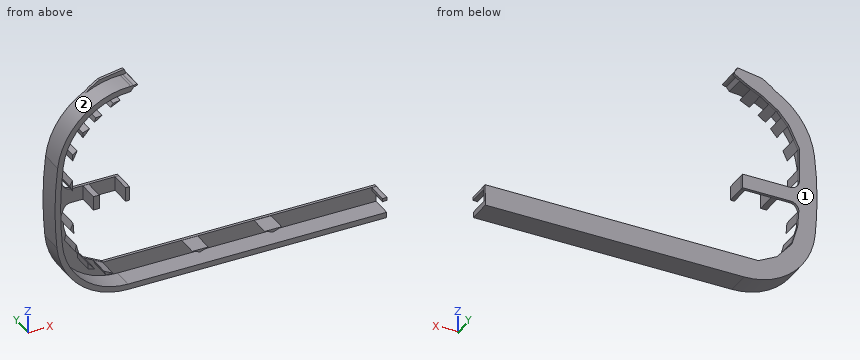
```python
from build123d import *

# Parameters (mm, degrees)
PAD356_DEPTH  = 12.5
PAD357_DEPTH  = 1.5
SKETCH835_W   = 2.131072
SKETCH835_H   = 7.619457
SKETCH835_W_2 = 3.147286
SKETCH835_H_2 = 7.516819
PAD359_DEPTH  = 11


with BuildPart() as part:
    # Sketch830 → Pad356 (new body)
    with BuildSketch(Plane.XZ):
        with BuildLine():
            Line((-1.478534, -110.025169), (137.370667, -110.025169))
            Line((137.370667, -107.025169), (137.370667, -110.025169))
            Line((-1.431571, -107.025169), (137.370667, -107.025169))
            ThreePointArc((-36.592097, -75.335952), (-25.110465, -97.94725), (-1.431571, -107.025169))
            ThreePointArc((-36.186878, -30.666211), (-37.587109, -52.990217), (-36.592097, -75.335952))
            ThreePointArc((0, 1.374966), (-24.161208, -7.792765), (-36.186878, -30.666211))
            Line((1.544739, 3.529825), (0, 1.374966))
            ThreePointArc((1.544739, 3.529825), (2.72516, 3.732882), (3.781105, 4.298219))
            Line((3.239563, 4.948117), (3.781105, 4.298219))
            ThreePointArc((1.508208, 4.37461), (2.420143, 4.521718), (3.239563, 4.948117))
            Line((0.022068, 4.37461), (1.508208, 4.37461))
            ThreePointArc((0.022068, 4.37461), (-26.243945, -5.630658), (-39.196845, -30.575221))
            ThreePointArc((-39.196845, -30.575221), (-40.587676, -52.998313), (-39.596378, -75.442618))
            ThreePointArc((-39.596378, -75.442618), (-27.212376, -100.091175), (-1.478534, -110.025169))
        make_face()
    extrude(amount=PAD356_DEPTH)

    # Sketch831 → Pad357 (join)
    with BuildSketch(Plane.XZ):
        with BuildLine():
            Line((-11.20697, 4.995917), (2.081055, 7.171183))
            Line((2.081055, 7.171183), (3.884949, 3.346928))
            Line((3.884949, 3.346928), (-3.071976, -0.758803))
            Line((-3.071976, -0.758803), (-10.956131, -4.609589))
            Line((-10.956131, -4.609589), (-19.896614, -10.750674))
            Line((-19.896614, -10.750674), (-25.51712, -17.174105))
            Line((-25.51712, -17.174105), (-31.174488, -28.94161))
            Line((-31.174488, -28.94161), (-31.174488, -40.845127))
            Line((-31.174488, -40.845127), (-31.174488, -47.004086))
            ThreePointArc((-31.174488, -47.004086), (-29.668559, -50.63972), (-26.032925, -52.145649))
            Line((-26.032925, -52.145649), (-0.596695, -52.145649))
            Line((-0.596695, -52.145649), (-0.596695, -59.85376))
            Line((-0.596695, -59.85376), (-26.454301, -59.85376))
            ThreePointArc((-26.454301, -59.85376), (-29.668775, -61.254046), (-30.832452, -64.561539))
            Line((-30.832452, -64.561539), (-30.207592, -73.162094))
            Line((-30.207592, -73.162094), (-27.154285, -83.944923))
            Line((-27.154285, -83.944923), (-18.964409, -93.499779))
            Line((-18.964409, -93.499779), (-9.168678, -98.558228))
            Line((-9.168678, -98.558228), (-2.331345, -98.558228))
            Line((-2.331345, -98.558228), (137.626465, -98.558228))
            Line((137.626465, -98.558228), (137.14772, -109.564461))
            Line((137.14772, -109.564461), (2.745987, -109.564461))
            Line((2.745987, -109.564461), (-3.35627, -109.564461))
            Line((-3.35627, -109.564461), (-8.527748, -108.903885))
            Line((-8.527748, -108.903885), (-14.660988, -106.811363))
            Line((-14.660988, -106.811363), (-18.737785, -105.296097))
            Line((-18.737785, -105.296097), (-23.031059, -102.842796))
            Line((-23.031059, -102.842796), (-25.966358, -100.308403))
            Line((-25.966358, -100.308403), (-29.71846, -96.772774))
            Line((-29.71846, -96.772774), (-33.867416, -91.108543))
            Line((-33.867416, -91.108543), (-35.409092, -87.704582))
            Line((-35.409092, -87.704582), (-37.577, -82.887016))
            Line((-37.577, -82.887016), (-39.02227, -76.142418))
            Line((-39.02227, -76.142418), (-39.504028, -68.916061))
            Line((-39.504028, -68.916061), (-39.795753, -62.945045))
            Line((-39.795753, -62.945045), (-39.795753, -54.118259))
            Line((-39.795753, -54.118259), (-39.795753, -44.679527))
            Line((-39.795753, -44.679527), (-38.558964, -32.354319))
            Line((-38.558964, -32.354319), (-38.395519, -29.4237))
            Line((-38.395519, -29.4237), (-36.619396, -22.319212))
            Line((-36.619396, -22.319212), (-33.174793, -14.730327))
            Line((-33.174793, -14.730327), (-28.806725, -8.890129))
            Line((-28.806725, -8.890129), (-22.724854, -3.669405))
            Line((-22.724854, -3.669405), (-15.835655, 1.92807))
            Line((-15.835655, 1.92807), (-11.20697, 4.995917))
        make_face()
    extrude(amount=PAD357_DEPTH)

    # Sketch835 → Pad359 (join)
    with BuildSketch(Plane.XZ.offset(1.5)):
        Polygon((-10.797218, -4.39096), (-5.61734, -1.866684), (-9.447662, -2.509944), align=None)
        Polygon((-19.402313, -10.356634), (-15.412445, -7.539076), (-18.804184, -8.036141), align=None)
        Polygon((-25.540901, -17.185297), (-22.080704, -13.161652), (-25.735592, -14.506651), align=None)
        Polygon((-28.749714, -23.759703), (-31.132679, -28.766081), (-31.176563, -25.309376), align=None)
        Polygon((-31.262688, -39.822292), (-31.262688, -45.629166), (-32.695404, -42.60001), align=None)
        with Locations((-1.667923, -55.987685)):
            Rectangle(SKETCH835_W, SKETCH835_H)
        with Locations((-18.408268, -55.977922)):
            Rectangle(SKETCH835_W_2, SKETCH835_H_2)
        Polygon((-30.88335, -63.977547), (-30.474003, -69.971565), (-32.403786, -67.427757), align=None)
        Polygon((-29.178089, -76.970978), (-27.78371, -82.030663), (-29.80479, -80.196259), align=None)
        Polygon((-23.049667, -88.872955), (-19.251656, -93.215378), (-22.826111, -92.215782), align=None)
        Polygon((-14.334663, -95.893806), (-9.420021, -98.582397), (-13.340538, -98.320648), align=None)
        Polygon((33.074181, -98.633934), (41.61673, -98.633934), (37.240623, -100.138222), align=None)
        Polygon((71.901031, -98.722458), (81.025146, -98.722458), (76.512283, -100.363495), align=None)
        Polygon((135.082978, -98.65696), (135.205872, -100.520859), (137.438461, -100.254593), (137.540878, -98.656967), align=None)
    extrude(amount=PAD359_DEPTH)


with BuildPart() as part_1:
    # Body024 placement: moved
    add(part.part.moved(Location((88, -111, 4))))


solid = part_1.part
```
Geometry check sheet. Reference: the model listing, model coordinates, mm. Face numbers are marked on the shaded views. A direction names the side the tool comes from. Coordinates: 2 decimals unless noted, no trailing zeros. Order: outer loops, then holes, each group sorted by start corner. A loop starts at its lowest first (then second) coordinate and runs counter-clockwise, first axis right, second up. Notation, with made-up numbers: (-25, 7) - (-19, 7) arc R21 cw to (-19, 41) - close; hole circle Ø9 at (-11, -6.5). An arc over 180 degrees is marked (long way). Answer in a Markdown table with one row per item. Add a question column.
1. Material ranges on L1, parallel to X at y = -117.5, z = -50; L2, parallel to Z at x = 72, y = -114.5; L3, parallel to Z at x = 90, y = -112.75, recorded low to high. Write a range as [from, to].
2. Access from +Z, -Z, +X, -X, +Y, -Y to the whole of each face (thin tool, end or side, straight path). Record for the marked faces 1 and 2.
3. Section check C-C (x = 186.5). Enter the section's corners in (y, z), plus the area to 3 significant figures.
4. Gauge pin test, flat ends, axial feed: pin 1 Ø0.8 at (x, y) = (69, -111.5) entering from +Z; pin 2 Ø2.5 at (y, z) = (-118.5, -53) entering from +X; pin 3 Ø0.8 at (y, z) = (-111.5, -31.5) entering from +X. Record the tip position at first contact, or that the pin passes through.
5. Section check A-A (y = -121.25). Give the number of separate pieces and of enclosed holes in the cut face, plus the area to 3 significant figures.
6. Section check B-B (x = 123.5). Enter the section's corners in (y, z), plus the area to 3 significant figures.
Data:
| question | item | result |
|---|---|---|
| 1 | L1 | x = [47.41, 50.41], [68.02, 71.17], [85.27, 87.4] |
| 1 | L2 | z = [-103.17, -99.9], [-3.95, -3.63], [1.67, 4.98] |
| 1 | L3 | z = [-106.03, -103.03], [7.56, 8.42] |
| 2 | face 1 | +Z, -Z, +X, -X, +Y |
| 2 | face 2 | +Z, -X, -Y |
| 3 | outline | (-123.5, -106.03) - (-111, -106.03) - (-111, -94.56) - (-112.5, -94.56) - (-112.5, -103.03) - (-123.5, -103.03) - close |
| 3 | area | 50.2 mm² |
| 4 | pin 1 | stops at z = 3.71 |
| 4 | pin 2 | stops at x = 87.4 |
| 4 | pin 3 | stops at x = 56.83 |
| 5 | separate pieces | 15 |
| 5 | enclosed holes | 0 |
| 5 | area | 982 mm² |
| 6 | outline | (-123.5, -106.03) - (-111, -106.03) - (-111, -94.56) - (-112.5, -94.56) - (-112.5, -94.63) - (-123.5, -94.63) - (-123.5, -95.51) - (-112.5, -95.51) - (-112.5, -103.03) - (-123.5, -103.03) - close |
| 6 | area | 59.8 mm² |
